Verification items for this drawing (mm, ordinates from the low corner). A direction names the side the tool comes from. Round coordinates to 2 decimals unless told otherwise and drop trailing zeros. Order: outer loops, then holes, each group sorted by start corner. A loop starts at its lowest first (then second) coordinate and runs counter-clockwise, first axis right, second up. Notation, with made-up numbers: M -32.5,72 L 26.5,72 A15 ccw 26.5,84 Z; hole C 38,71 d7. An arc over 180 degrees is marked long. Return JSON: item names as keys, results as strings. Group by question number.
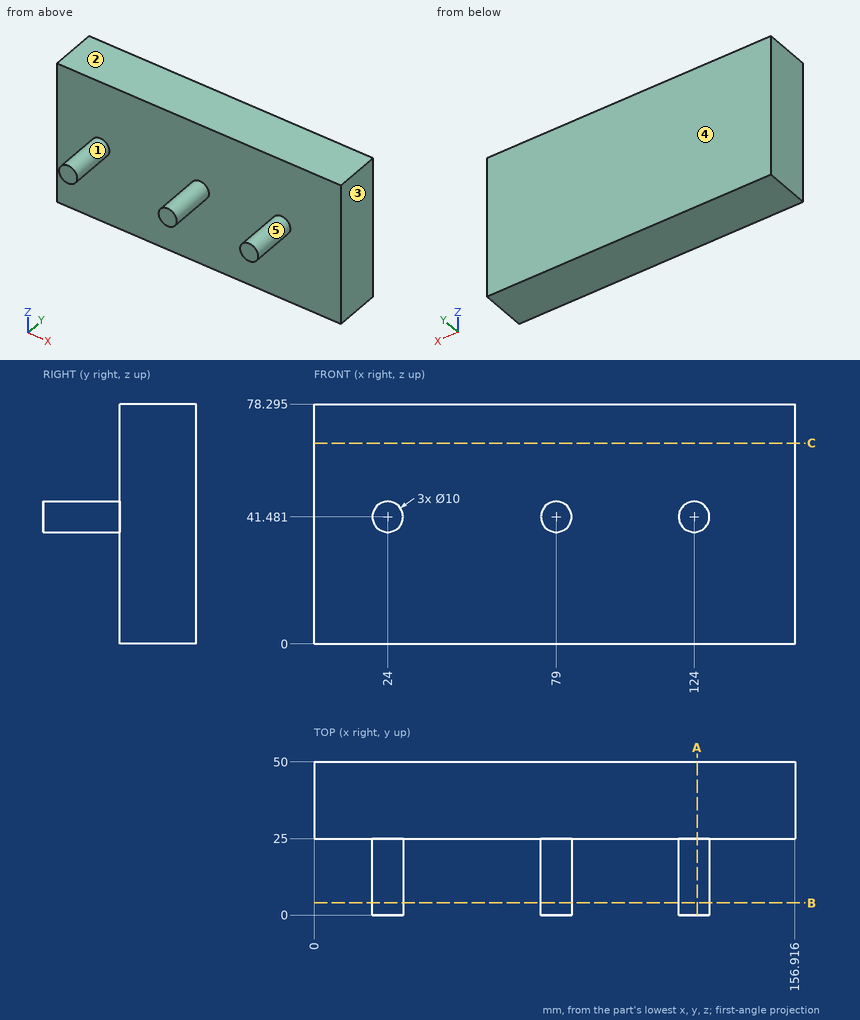
1. Draft check along X on the marked faces 1, 2 and 3. Enter one of: +X half, -X half, draft (parallel to the pull), parting line (faces both ways), or undercut.
2. Cross-section at A-A (x = 125). Enter the section's corners in (y, z) (1 decimal), plus the area to 3 significant figures.
3. Access from +Z, -Z, +X, -X, +Y, -Y to the whole of each face (thin tool, end or side, straight path). Record for the marked faces 4 and 5.
4. Cross-section at B-B (y = 4). Enter the section's corners in (x, z), plus the area to 3 significant figures.
5. Go/stop test with flat-tipped pins: pin 1 (3 mm diameter, centred on x = 81.5, y = 11.5, fed in from -Z); pin 2 (2 mm diameter, centred on y = 29.5, z = 23.5, fed in from -X); pin 3 (1.5 mm diameter, centred on x = 22.5, z = 60.5, fed in from -Y). Record where each tip stops, or that it passes through.
6. Thickness scan on line 1 along X through (y, z) = (20.5, 42); line 2 along X through (y, z) = (12, 40.5); line 3 along Y through (x, z) = (8, 72.5). Record the ranges inside material, lowest first. Write a range as from..to.
7. Cross-section at C-C (z = 65.5). Enter the section's corners in (x, y).
Computed:
{
 "1": {"face 1": "undercut", "face 2": "draft", "face 3": "+X half"},
 "2": {"outline": "M 0,36.6 L 25,36.6 L 25,0 L 50,0 L 50,78.3 L 25,78.3 L 25,46.4 L 0,46.4 Z", "area": "2,200 mm²"},
 "3": {"face 4": "+Z, -Z, +X, -X, +Y", "face 5": "-Y"},
 "4": {"outline": "C 24,41.48 d10; C 79,41.48 d10; C 124,41.48 d10", "area": "236 mm²"},
 "5": {"pin 1": "stops at z = 36.58", "pin 2": "stops at x = 0", "pin 3": "stops at y = 25"},
 "6": {"line 1": "x = 19.03..28.97, 74.03..83.97, 119.03..128.97", "line 2": "x = 19.1..28.9, 74.1..83.9, 119.1..128.9", "line 3": "y = 25..50"},
 "7": {"outline": "M 0,25 L 156.92,25 L 156.92,50 L 0,50 Z"}
}
